Work out the finished part from the listing and answer in its coordinate system (mm). A direction names the side the tool comes from. Coordinates: 2 decimals unless noted, no trailing zeros. Loops run counter-clockwise (first coordinate to the right, second up) from the corner with the lowest first, then second, coordinate; pieces in that order, holes last. Notation, with made-up numbers: (-2, 75.5) -> (38, 75.5) arc R12 ccw to (38, 84.5) -> close; hole circle Ø8 at (-3, -31.5). An arc over 180 degrees is marked (long way). One line per question, with ' | ' between items.
```python
from build123d import *

# Parameters (mm, degrees)
SKETCH1_R               = 32.5
BOSS_EXTRUDE1_DEPTH     = 25
CUT_EXTRUDE1_DEPTH      = 5
CUT_EXTRUDE2_DEPTH      = 82.699111815
CUT_EXTRUDE2_DEPTH_BACK = 82.699111815
SKETCH3_R               = 2.5


with BuildPart() as part:
    # Sketch1 → Boss-Extrude1 (new body)
    with BuildSketch(Plane(origin=(0, 0, 0), x_dir=(1, 0, 0), z_dir=(0, 1, 0))):
        with BuildLine():
            Line((-22.5, -35), (22.5, -35))
            Line((22.5, -35), (22.5, -49.494897428))
            Line((22.5, -49.494897428), (25, -49.494897428))
            Line((25, -49.494897428), (25, -35))
            Line((25, -35), (25, -24.494897428))
            ThreePointArc((25, -24.494897428), (33.886456264, 8.758315013), (10, 33.541019662))
            Line((10, 33.541019662), (10, 38.541019662))
            Line((10, 38.541019662), (-10, 38.541019662))
            Line((-10, 38.541019662), (-10, 33.541019662))
            ThreePointArc((-10, 33.541019662), (-33.886456264, 8.758315013), (-25, -24.494897428))
            Line((-25, -24.494897428), (-25, -35))
            Line((-25, -35), (-25, -49.494897428))
            Line((-25, -49.494897428), (-22.5, -49.494897428))
            Line((-22.5, -49.494897428), (-22.5, -35))
        make_face()
        with Locations(Location((0, 0, 0), (0, 0, 270))):
            Circle(SKETCH1_R, mode=Mode.SUBTRACT)
        with BuildLine():
            Line((-22.5, -26.809513237), (-22.5, -32.5))
            Line((-22.5, -32.5), (-12.990381057, -32.5))
            ThreePointArc((-12.990381057, -32.5), (-17.971844557, -30.033527985), (-22.5, -26.809513237))
        make_face(mode=Mode.SUBTRACT)
        with BuildLine():
            Line((22.5, -32.5), (22.5, -26.809513237))
            ThreePointArc((22.5, -26.809513237), (17.971844557, -30.033527985), (12.990381057, -32.5))
            Line((12.990381057, -32.5), (22.5, -32.5))
        make_face(mode=Mode.SUBTRACT)
    extrude(amount=BOSS_EXTRUDE1_DEPTH)

    # Sketch2 → Cut-Extrude1 (cut)
    with BuildSketch(Plane(origin=(0, 0, -38.541019662), x_dir=(-1, 0, 0), z_dir=(0, 0, -1))):
        Polygon((-6.380534686, 25), (5.277156767, 0), (6.380534686, 0), (-5.277156767, 25), align=None)
        Polygon((-1.967023011, 25), (10, 25), (10, 0), (9.690668443, 0), align=None)
        Polygon((-9.690668443, 25), (-10, 25), (-10, -0.029833576), (1.967023011, 0), align=None)
    extrude(amount=-CUT_EXTRUDE1_DEPTH, mode=Mode.SUBTRACT)

    # Sketch3 → Cut-Extrude2 (cut, two sides: drawn at the far end of the back side and taken through both)
    with BuildSketch(Plane(origin=(25, 0, 0), x_dir=(0, 0, -1), z_dir=(1, 0, 0)).offset(-CUT_EXTRUDE2_DEPTH_BACK)):
        with Locations((-44.494897428, 12.5)):
            Circle(SKETCH3_R)
    extrude(amount=CUT_EXTRUDE2_DEPTH + CUT_EXTRUDE2_DEPTH_BACK, mode=Mode.SUBTRACT)


solid = part.part
```
1) The mould has two halves that part along X. Classify faces 6 (the face through (24, 12, 49.495)), 7 (the face through (-3.943, 12.325, -36.076)), 8 (the face through (18.039, 12.325, 29.993)): released by +X, released by -X, zero draft, split by the parting line, or undercut.
Check values:
face 6: zero draft | face 7: released by -X | face 8: undercut
2) Flat-ended cylindrical pins translate along their axes: pin 1 (1 mm diameter, centred on x = -15, y = 10.5, fed in from -Z); pin 2 (1.5 mm diameter, centred on y = 12.5, z = -26.5, fed in from +X); pin 3 (6.5 mm diameter, centred on y = 12.5, z = 44.49, fed in from -X). Find the tip coordinate at first contact, or state that the pin passes through.
Check values:
pin 1: stops at z = -31.86 | pin 2: stops at x = 23.71 | pin 3: stops at x = -25
3) For faces 1 (the face through (22.5, 12, 41)), 2 (the face through (25, 12, 37)), 3 (the face through (3.78, 12.32, -36.08)), 4 (the face through (-5, 15, -33.541)), 5 (the face through (-25, 12, 37)), determine the directions among +Z, -Z, +X, -X, +Y, -Y from which every point of the face is accessible in a straight line to the end or side of a thin tool.
Check values:
face 1: +Z, +Y, -Y | face 2: +Z, +X, +Y, -Y | face 3: -Z, +X, -Y | face 4: -Z, -X, +Y | face 5: +Z, -X, +Y, -Y
4) Find section B-B (y = 12.5). State how many separate pieces and enclosed holes the cut face has, plus the area to 3 significant figures.
Check values:
separate pieces: 3 | enclosed holes: 3 | area: 707 mm^2
5) Find section A-A (z = 0). Write down the section's boundary in (x, y), plus the area to 3 significant figures.
Check values:
outline: (-35, 0) -> (-32.5, 0) -> (-32.5, 25) -> (-35, 25) -> close; (32.5, 0) -> (35, 0) -> (35, 25) -> (32.5, 25) -> close | area: 125 mm^2
6) Find section C-C (x = 0). Write down the section's boundary in (y, z).
Check values:
outline: (0, -33.54) -> (4.22, -33.54) -> (4.22, -38.54) -> (11.32, -38.54) -> (11.32, -33.54) -> (13.68, -33.54) -> (13.68, -38.54) -> (20.78, -38.54) -> (20.78, -33.54) -> (25, -33.54) -> (25, -32.5) -> (0, -32.5) -> close; (0, 32.5) -> (25, 32.5) -> (25, 35) -> (0, 35) -> close
7) Find section D-D (y = 2.75). Write down the section's boundary in (x, z).
Check values:
outline: (-25, 24.49) arc R35 ccw to (-10, -33.54) -> (-8.41, -33.54) -> (-8.41, -38.54) -> (-5.1, -38.54) -> (-5.1, -33.54) -> (-3.99, -33.54) -> (-3.99, -38.54) -> (-0.68, -38.54) -> (-0.68, -33.54) -> (10, -33.54) arc R35 ccw to (25, 24.49) -> (25, 49.49) -> (22.5, 49.49) -> (22.5, 35) -> (-22.5, 35) -> (-22.5, 49.49) -> (-25, 49.49) -> close; hole circle Ø65 at (0, 0); hole (-22.5, 26.81) arc R35 cw to (-12.99, 32.5) -> (-22.5, 32.5) -> close; hole (12.99, 32.5) arc R35 cw to (22.5, 26.81) -> (22.5, 32.5) -> close
8) Find the intervals of material crossed by line 1 along Z through (x, y) = (24.4, 12.5); line 2 along X through (y, z) = (20.25, 45.5); line 3 along X through (y, z) = (6.25, 27), in increasing order.
Check values:
line 1: z = -25.09 to -21.47, 21.47 to 41.99, 46.99 to 49.49 | line 2: x = -25 to -22.5, 22.5 to 25 | line 3: x = -25 to -22.5, -22.27 to -18.09, 18.09 to 22.27, 22.5 to 25
